Source: CAD feature listing. Evaluate the final solid. Frame: model axes, mm. A direction names the side the tool comes from. Give positions to 0.01 mm unless a question says otherwise; leave off trailing zeros. Loops run counter-clockwise (first coordinate to the right, second up) from the corner with the lowest first, then second, coordinate; pieces in that order, holes last. Notation, with made-up numbers: (-1.75, 39.5) - (28.25, 39.5) arc R27 ccw to (28.25, 65.5) - close; hole circle Ø2 at (-26.5, 49.5). An arc over 180 degrees is marked (long way). Write each question's results on one line, items separated by ' | '. Start each with the question number.
(1) Contact query for flat-ended pins moving along their axis: pin 1 (2 mm diameter, centred on x = -1, y = -12, fed in from -Z); pin 2 (7 mm diameter, centred on x = 0, y = 47, fed in from +Z); pin 3 (3 mm diameter, centred on x = -13, y = 0, fed in from -Z); pin 4 (6 mm diameter, centred on x = -12, y = 47, fed in from -Z). Output: stop coordinate, or through.
(2) Material intervals for line 1 along X through (y, z) = (47, 3.05); line 2 along Y through (x, z) = (0, 3.8); line 3 along Y through (x, z) = (0, 0.8), sorted ascending. Write a range as [from, to].
(3) Pull-direction query (Y, two-part tool) for faces 1 (the cylindrical face through (0.38, -39.5, 4.93)), 2 (the flat face through (-25, 10, 5)), 3 (the cylindrical face through (-13.2, -33.7, 8)); classes: pulls with the +Y half, pulls with the -Y half, needs draft (parallel to the pull), parting line crosses it, or undercut.
(4) Cut plane A-A on y = 47. Return the cut outline in (x, z), then the cut area to 4 significant figures.
(5) Reachability of faces 4 (the cylindrical face through (4.38, -8.43, 3.45)), 5 (the cylindrical face through (14.187, -33.344, 8.028)), 6 (the cylindrical face through (-9.753, 0.143, 0.986)), 7 (the flat face through (0, 50, 1)) from +Z, -Z, +X, -X, +Y, -Y: full face, straight path, thin tool, end or side. Return the list, or none.
(6) Cut plane B-B on y = -13. Return the cut outline in (x, z), then the cut area to 3 significant figures.
(7) Cut plane D-D on z = 4.5. Give the number of separate pieces and of enclosed holes in the cut face, then the cut area to 3 significant figures.
(8) Cut plane C-C on x = -6. Return the cut outline in (y, z).
from build123d import *

# Parameters (mm, degrees)
SKETCH_1_R          = 2.25
SKETCH_1_R_2        = 9.5
SKETCH_1_R_3        = 1.75
EXTRUDE_1_DEPTH     = 10
SKETCH_3_R          = 16
CUT_EXTRUDE_1_DEPTH = 3
SKETCH_4_R          = 4
CUT_EXTRUDE_2_DEPTH = 4
SKETCH_5_W          = 50
SKETCH_5_H          = 10
CUT_EXTRUDE_3_DEPTH = 1
SKETCH_6_R          = 3.25
CUT_EXTRUDE_4_DEPTH = 2


with BuildPart() as part:
    # 스케치1 → 보스-돌출1 (new body)
    with BuildSketch(Plane.XY):
        with BuildLine():
            Line((-25, 0), (-25, 52))
            Line((-25, 52), (25, 52))
            Line((25, 52), (25, -30.581857367))
            ThreePointArc((25, -30.581857367), (0, -39.5), (-25, -30.581857367))
            Line((-25, -30.581857367), (-25, 0))
        make_face()
        with Locations((-12.341540694, -29.795114923)):
            Circle(SKETCH_1_R, mode=Mode.SUBTRACT)
        with Locations((12.341540694, -29.795114923)):
            Circle(SKETCH_1_R, mode=Mode.SUBTRACT)
        with Locations((0, 47)):
            Circle(SKETCH_1_R, mode=Mode.SUBTRACT)
        with Locations((12, 47)):
            Circle(SKETCH_1_R, mode=Mode.SUBTRACT)
        with Locations((-12, 47)):
            Circle(SKETCH_1_R, mode=Mode.SUBTRACT)
        Circle(SKETCH_1_R_2, mode=Mode.SUBTRACT)
        with Locations((-13, 0)):
            Circle(SKETCH_1_R_3, mode=Mode.SUBTRACT)
        with Locations((0, 13)):
            Circle(SKETCH_1_R_3, mode=Mode.SUBTRACT)
        with Locations((13, 0)):
            Circle(SKETCH_1_R_3, mode=Mode.SUBTRACT)
        with Locations((0, -13)):
            Circle(SKETCH_1_R_3, mode=Mode.SUBTRACT)
    extrude(amount=EXTRUDE_1_DEPTH)

    # 스케치3 → 컷-돌출1 (cut)
    with BuildSketch(Plane.XY.offset(10)):
        Circle(SKETCH_3_R)
    extrude(amount=-CUT_EXTRUDE_1_DEPTH, mode=Mode.SUBTRACT)

    # 스케치4 → 컷-돌출2 (cut)
    with BuildSketch(Plane.XY.offset(10)):
        with Locations((-12, 47)):
            Circle(SKETCH_4_R)
        with Locations((0, 47)):
            Circle(SKETCH_4_R)
        with Locations((12, 47)):
            Circle(SKETCH_4_R)
        with Locations((12.341540694, -29.795114923)):
            Circle(SKETCH_4_R)
        with Locations((-12.341540694, -29.795114923)):
            Circle(SKETCH_4_R)
    extrude(amount=-CUT_EXTRUDE_2_DEPTH, mode=Mode.SUBTRACT)

    # 스케치5 → 컷-돌출3 (cut)
    with BuildSketch(Plane(origin=(0, 0, 0), x_dir=(-1, 0, 0), z_dir=(0, 0, -1))):
        with Locations((0, 47)):
            Rectangle(SKETCH_5_W, SKETCH_5_H)
    extrude(amount=-CUT_EXTRUDE_3_DEPTH, mode=Mode.SUBTRACT)

    # 스케치6 → 컷-돌출4 (cut)
    with BuildSketch(Plane(origin=(0, 0, 0), x_dir=(-1, 0, 0), z_dir=(0, 0, -1))):
        with Locations((0, 13)):
            Circle(SKETCH_6_R)
        with Locations((13, 0)):
            Circle(SKETCH_6_R)
        with Locations((0, -13)):
            Circle(SKETCH_6_R)
        with Locations((-13, 0)):
            Circle(SKETCH_6_R)
    extrude(amount=-CUT_EXTRUDE_4_DEPTH, mode=Mode.SUBTRACT)


solid = part.part
Ans:
1) pin 1: z = 2 | pin 2: z = 6 | pin 3: through | pin 4: z = 1
2) line 1: [-25, -14.25], [-9.75, -2.25], [2.25, 9.75], [14.25, 25] | line 2: [-39.5, -14.75], [-11.25, -9.5], [9.5, 11.25], [14.75, 44.75], [49.25, 52] | line 3: [-39.5, -16.25], [-9.75, -9.5], [9.5, 9.75], [16.25, 42]
3) face 1: pulls with the -Y half | face 2: needs draft | face 3: undercut
4) outline: (-25, 1) - (-14.25, 1) - (-14.25, 6) - (-16, 6) - (-16, 10) - (-25, 10) - close; (-9.75, 1) - (-2.25, 1) - (-2.25, 6) - (-4, 6) - (-4, 10) - (-8, 10) - (-8, 6) - (-9.75, 6) - close; (2.25, 1) - (9.75, 1) - (9.75, 6) - (8, 6) - (8, 10) - (4, 10) - (4, 6) - (2.25, 6) - close; (14.25, 1) - (25, 1) - (25, 10) - (16, 10) - (16, 6) - (14.25, 6) - close | area: 286.5 mm^2
5) face 4: +Z, -Z | face 5: +Z | face 6: -Z | face 7: -Z, +X, -X, +Y
6) outline: (-25, 0) - (-3.25, 0) - (-3.25, 2) - (-1.75, 2) - (-1.75, 7) - (-9.33, 7) - (-9.33, 10) - (-25, 10) - close; (1.75, 2) - (3.25, 2) - (3.25, 0) - (25, 0) - (25, 10) - (9.33, 10) - (9.33, 7) - (1.75, 7) - close | area: 414 mm^2
7) separate pieces: 1 | enclosed holes: 10 | area: 4,030 mm^2
8) outline: (-39.04, 0) - (-7.37, 0) - (-7.37, 7) - (-14.83, 7) - (-14.83, 10) - (-39.04, 10) - close; (7.37, 0) - (42, 0) - (42, 1) - (52, 1) - (52, 10) - (14.83, 10) - (14.83, 7) - (7.37, 7) - close
